Design review of the part shown in the three views and the two pictorial views. Dimensions are in mm from the part's minimum x, y and z. A direction names the side the tool comes from. Coordinates: 2 decimals unless noted, no trailing zeros. Order: outer loops, then holes, each group sorted by start corner. A loop starts at its lowest first (then second) coordinate and runs counter-clockwise, first axis right, second up. Notation, with made-up numbers: (-22.75, 8) -> (31.25, 8) arc R26 ccw to (31.25, 44) -> close; hole circle Ø6 at (39, 83.25). An arc over 180 degrees is marked (long way). Write item = value, one per line. Start each with the question number.
1) Wall thickness on probe 1 along X at (y, z) = (4, 3.4); probe 2 along X at (y, z) = (4, 1.2); probe 3 along Y at (x, z) = (8.25, 5.3): over which ranges is each line inside the solid? List them lowest first. Write a range as [from, to].
2) Machinability: for the marked faces 1, 2 and 3, which of the approach directions +Z, -Z, +X, -X, +Y, -Y give a long, thin tool a straight path to every point of the face, cutting with its end or side? Answer none if there is none.
3) Consider section B-B on y = 3. Give the boundary of the cut face in (x, z), and give its area (3 significant figures).
4) Consider section A-A on x = 7.75. Give the boundary of the cut face in (y, z), and give its area (3 significant figures).
5) Draft analysis for pull direction Z (two halves, no side actions). For the marked faces 4, 5 and 6, state which applies: +Z half, -Z half, draft (parallel to the pull), parting line (faces both ways), or undercut.
6) Consider section C-C on x = 0.5. Give the boundary of the cut face in (y, z).
7) Insertion check: pin 1 Ø1.5 at (x, z) = (2, 2.5) entering from -Y; pin 2 Ø1.5 at (y, z) = (2.5, 3.5) entering from +X; pin 3 Ø3 at (x, y) = (1, 3.5) entering from +Z. Each pin has a flat end and moves straight along its axis. Give the tip position at first contact, or say it passes through.
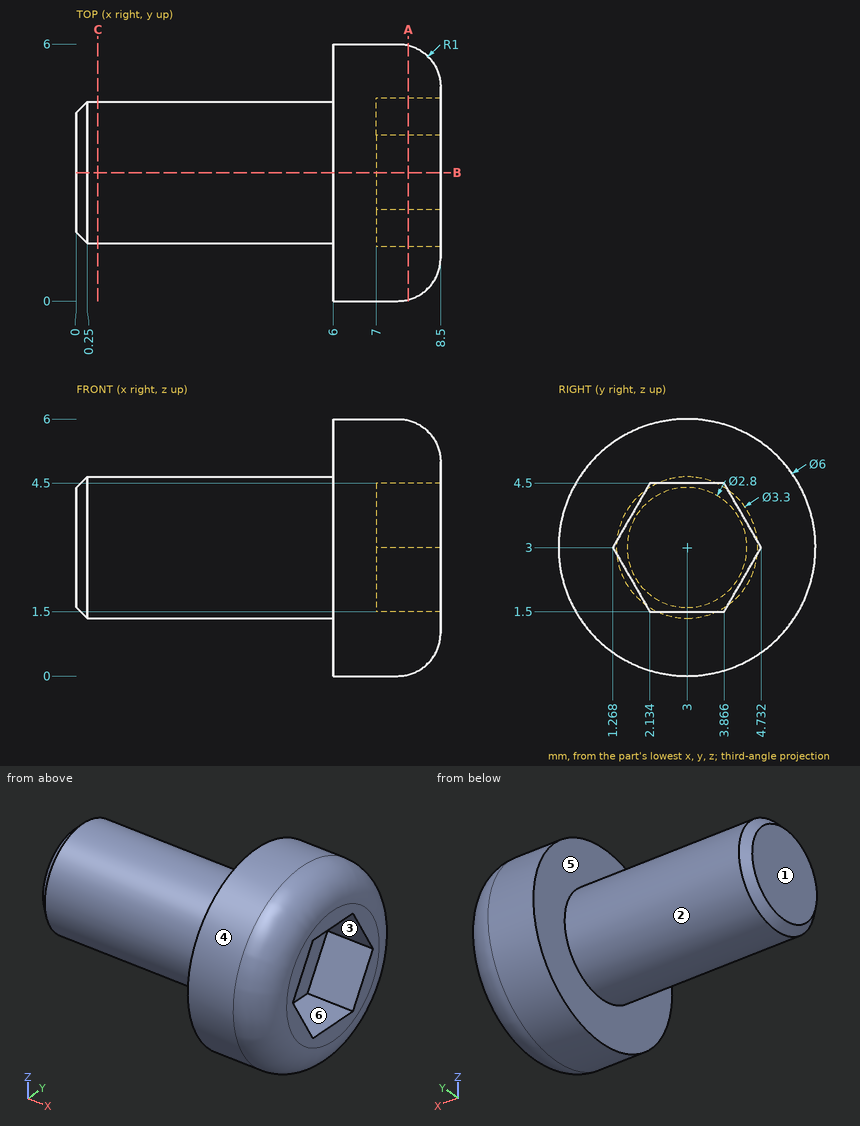
Answer sheet:
q1.probe_1 = [0, 7]
q1.probe_2 = [6, 8.5]
q1.probe_3 = [1.66, 4.34]
q2.face_1 = +Z, -Z, -X, +Y, -Y
q2.face_2 = -X
q2.face_3 = +X
q3.outline = (0, 1.6) -> (0.25, 1.35) -> (6, 1.35) -> (6, 0) -> (7.5, 0) arc R1 ccw to (8.5, 1) -> (8.5, 1.5) -> (7, 1.5) -> (7, 4.5) -> (8.5, 4.5) -> (8.5, 5) arc R1 ccw to (7.5, 6) -> (6, 6) -> (6, 4.65) -> (0.25, 4.65) -> (0, 4.4) -> close
q3.area = 29.8 mm2
q4.outline = circle Ø5.94 at (3, 3); hole (1.27, 3) -> (2.13, 1.5) -> (3.87, 1.5) -> (4.73, 3) -> (3.87, 4.5) -> (2.13, 4.5) -> close
q4.area = 19.9 mm2
q5.face_4 = parting line
q5.face_5 = draft
q5.face_6 = undercut
q6.outline = circle Ø3.3 at (3, 3)
q7.pin_1 = 1.35
q7.pin_2 = 7
q7.pin_3 = 4.65
